For this review, take the finished solid that the model builds, in its own axes (mm). A direction names the side the tool comes from. Round coordinates to 2 decimals unless told otherwise and drop trailing zeros. Loops run counter-clockwise (first coordinate to the right, second up) from the corner with the lowest first, then second, coordinate; pieces in that order, holes last. Notation, with made-up numbers: M 85,-19 L 92,-19 A21 ccw 92,8 Z; hole C -20,-22.75 d2. An arc over 180 degrees is marked long. One line per question, with ' | ' between items. Start each with the question number.
1) For probe 1 along Z at (x, y) = (12.5, -78); probe 2 along X at (y, z) = (-47, -13.5); probe 3 along Z at (x, y) = (29.15, -15.24), list the stretches that pass through material, from the lowest coordinate up. Write a range as from..to.
2) For pin 1 Ø1.1 at (x, y) = (1, -43.5) entering from +Z; pin 2 Ø3 at (y, z) = (-70, -25.5) entering from +X; pin 3 Ø3 at (x, z) = (15.5, 2) entering from -Y; pin 4 Ø13.5 at (x, y) = (18.5, -23) entering from -Z, all flat-tipped, find the tip position at first contact; note any pin that passes through.
3) We need section B-B (y = -15.24). Give the boundary of the cut face in (x, z).
4) We need section D-D (y = -70). Give the boundary of the cut face in (x, z), and give its area (3 significant figures).
5) We need section C-C (z = -7). Give the boundary of the cut face in (x, y).
6) Mouldability with a two-part tool opening along X and no side actions: class faces 1 (the face through (2, -36, 0)), 2 (the face through (27.394, -29, -12)), 3 (the face through (28.194, -68, -26)) as pulls with the +X half, pulls with the -X half, needs draft (parallel to the pull), parting line crosses it, or undercut.
7) We need section A-A (y = -52). Give the boundary of the cut face in (x, z), and give its area (3 significant figures).
8) For faces 4 (the face through (29.78, -59.84, -12.36)), 5 (the face through (29.33, -2.85, -21.12)), 6 (the face through (15, -61.345, -12)), 7 (the face through (15, -57.535, -13)), 8 (the face through (16, -88.015, 2)), list the 3-axis set-ups (+Z, -Z, +X, -X, +Y, -Y) from which the entire face can be reached by the end or side of a thin tool; tool diameter is ignored.
```python
from build123d import *

# Parameters (mm, degrees)
BOSS_EXTRUDE1_DEPTH         = 3.81
SKETCH2_W                   = 27.394147034
SKETCH2_H                   = 24.384
BOSS_EXTRUDE2_DEPTH         = 3.81
SKETCH7_W                   = 24.13
SKETCH7_H                   = 61.344873393
BOSS_EXTRUDE3_DEPTH         = 3.81
FILLET1_R                   = 10
FILLET2_R                   = 10
FILLET3_R                   = 5
FILLET4_R                   = 5
SKETCH8_W                   = 24.384
SKETCH8_H                   = 30.48
BOSS_EXTRUDE4_DEPTH         = 3.81
FILLET5_R                   = 5
FILLET6_R                   = 10
FILLET8_R                   = 10
SKETCH9_W                   = 24.384
SKETCH9_H                   = 30.48
BOSS_EXTRUDE5_DEPTH         = 3.81
FILLET9_R                   = 10
FILLET10_R                  = 10
FILLET11_R                  = 5
F_1_4_0_25_DIAMETER_HOLE1_D = 6.35


with BuildPart() as part:
    # Sketch1 → Boss-Extrude1 (new body)
    with BuildSketch(Plane(origin=(0, 0, 0), x_dir=(0, 0, -1), z_dir=(1, 0, 0))):
        with BuildLine():
            Line((10, 0), (14.384, 0))
            ThreePointArc((14.384, 0), (21.455067812, -2.928932188), (24.384, -10))
            Line((24.384, -10), (24.384, -57.534873393))
            Line((24.384, -57.534873393), (0, -57.534873393))
            Line((0, -57.534873393), (0, -10))
            ThreePointArc((0, -10), (2.928932188, -2.928932188), (10, 0))
        make_face()
    extrude(amount=BOSS_EXTRUDE1_DEPTH)

    # Sketch2 → Boss-Extrude2 (add)
    with BuildSketch(Plane(origin=(0, -57.534873393, 0), x_dir=(-1, 0, 0), z_dir=(0, -1, 0))):
        with Locations((-13.697073517, 12.192)):
            Rectangle(SKETCH2_W, SKETCH2_H)
    extrude(amount=BOSS_EXTRUDE2_DEPTH)

    # Sketch7 → Boss-Extrude3 (add)
    with BuildSketch(Plane(origin=(27.394147034, 0, 0), x_dir=(0, 0, -1), z_dir=(1, 0, 0))):
        with Locations((12.065, -30.672436697)):
            Rectangle(SKETCH7_W, SKETCH7_H)
    extrude(amount=BOSS_EXTRUDE3_DEPTH)

    # Fillet1
    fillet1_edges = [part.edges().sort_by_distance(p)[0] for p in [
        (29.299147034, 0, -24.13),
    ]]
    fillet(fillet1_edges, radius=FILLET1_R)

    # Fillet2
    fillet2_edges = [part.edges().sort_by_distance(p)[0] for p in [
        (29.299147034, 0, 0),
    ]]
    fillet(fillet2_edges, radius=FILLET2_R)

    # Fillet3
    fillet3_edges = [part.edges().sort_by_distance(p)[0] for p in [
        (31.204147034, -61.344873393, -12.065),
    ]]
    fillet(fillet3_edges, radius=FILLET3_R)

    # Fillet4
    fillet4_edges = [part.edges().sort_by_distance(p)[0] for p in [
        (0, -61.344873393, -12.192),
    ]]
    fillet(fillet4_edges, radius=FILLET4_R)

    # Sketch8 → Boss-Extrude4 (add)
    with BuildSketch(Plane(origin=(0, 0, -24.384), x_dir=(-1, 0, 0), z_dir=(0, 0, -1))):
        with Locations((-16.002, -72.933007505)):
            Rectangle(SKETCH8_W, SKETCH8_H)
    extrude(amount=BOSS_EXTRUDE4_DEPTH)

    # Fillet5
    # the kernel refuses this fillet: 5 mm, written as the material it takes off along each edge
    with BuildSketch(Plane(origin=(-8.330814429, -57.693007505, -28.194), x_dir=(0, 0, 1), z_dir=(1, 0, 0))) as fillet5_piece_1:
        with BuildLine():
            CenterArc((5, 4.856325772), FILLET5_R, 180, 76.231471248)
            Line((0, 4.856325772), (-0.1, 4.856325772))
            Line((-0.1, 4.856325772), (-0.1, 0))
            Line((-0.1, 0), (0, -0.1))
            ThreePointArc((0, -0.1), (1.905, -0.1), (3.7862, -0.097126515))
            Line((3.7862, -0.097126515), (3.81, 0))
        make_face()
    extrude(amount=48.665628858, mode=Mode.SUBTRACT)

    # Fillet6
    fillet6_edges = [part.edges().sort_by_distance(p)[0] for p in [
        (3.81, -88.173007505, -26.289),
    ]]
    fillet(fillet6_edges, radius=FILLET6_R)

    # Fillet8
    fillet8_edges = [part.edges().sort_by_distance(p)[0] for p in [
        (28.194, -88.173007505, -26.289),
    ]]
    fillet(fillet8_edges, radius=FILLET8_R)

    # Sketch9 → Boss-Extrude5 (add)
    with BuildSketch(Plane.XY):
        with Locations((16.002, -72.774873393)):
            Rectangle(SKETCH9_W, SKETCH9_H)
    extrude(amount=BOSS_EXTRUDE5_DEPTH)

    # Fillet9
    fillet9_edges = [part.edges().sort_by_distance(p)[0] for p in [
        (3.81, -88.014873393, 1.905),
    ]]
    fillet(fillet9_edges, radius=FILLET9_R)

    # Fillet10
    fillet10_edges = [part.edges().sort_by_distance(p)[0] for p in [
        (28.194, -88.014873393, 1.905),
    ]]
    fillet(fillet10_edges, radius=FILLET10_R)

    # Fillet11
    # the kernel refuses this fillet: 5 mm, written as the material it takes off along each edge
    with BuildSketch(Plane(origin=(3.81, -57.534873393, 3.81), x_dir=(0, -1, 0), z_dir=(1, 0, 0))) as fillet11_piece_1_section:
        with BuildLine():
            CenterArc((FILLET11_R, FILLET11_R), FILLET11_R, 180, 90)
            Line((0, FILLET11_R), (0, 0))
            Line((0, 0), (FILLET11_R, 0))
        make_face()
    fillet11_piece_1 = extrude(amount=36.884, mode=Mode.PRIVATE)
    fillet11_piece_1 = split(fillet11_piece_1, bisect_by=Plane(origin=(27.394147034, -58.779272815, 2.781917075), z_dir=(-1, 0, 0)), keep=Keep.TOP, mode=Mode.PRIVATE)
    add(fillet11_piece_1, mode=Mode.SUBTRACT)
    with BuildSketch(Plane(origin=(-8.69, -57.534873393, 3.81), x_dir=(0, -1, 0), z_dir=(1, 0, 0))) as fillet11_piece_2_section:
        with BuildLine():
            CenterArc((FILLET11_R, FILLET11_R), FILLET11_R, 180, 90)
            Line((0, FILLET11_R), (0, 0))
            Line((0, 0), (FILLET11_R, 0))
        make_face()
    fillet11_piece_2 = extrude(amount=49.384, mode=Mode.PRIVATE)
    fillet11_piece_2 = split(fillet11_piece_2, bisect_by=Plane(origin=(27.831342884, -61.431899575, 0), z_dir=(0, 0, 1)), keep=Keep.TOP, mode=Mode.PRIVATE)
    add(fillet11_piece_2, mode=Mode.SUBTRACT)

    # 1/4 (0.25) Diameter Hole1 (through all)
    with Locations(Plane(origin=(0, -15.24, -12.192), x_dir=(0, 0, -1), z_dir=(-1, 0, 0))):
        with Locations((0, 0)):
            Hole(F_1_4_0_25_DIAMETER_HOLE1_D / 2)


solid = part.part
```
Answers below:
1) probe 1: -28.19..-24.38, 0..3.81 | probe 2: 0..3.81, 27.39..31.2 | probe 3: -24.13..-15.37, -9.02..0
2) pin 1: z = 0 | pin 2: x = 28.19 | pin 3: y = -88.01 | pin 4: through
3) outline: M 0,-24.38 L 3.81,-24.38 L 3.81,-15.37 L 0,-15.37 Z; M 0,-9.02 L 3.81,-9.02 L 3.81,0 L 0,0 Z; M 27.39,-24.13 L 31.2,-24.13 L 31.2,-15.37 L 27.39,-15.37 Z; M 27.39,-9.02 L 31.2,-9.02 L 31.2,0 L 27.39,0 Z
4) outline: M 3.81,-28.19 L 28.19,-28.19 L 28.19,-24.38 L 3.81,-24.38 Z; M 3.81,0 L 28.19,0 L 28.19,3.81 L 3.81,3.81 Z | area: 186 mm^2
5) outline: M 0,-56.34 A5 ccw 5,-61.34 L 26.2,-61.34 A5 ccw 31.2,-56.34 L 31.2,-0.46 L 27.39,-0.46 L 27.39,-57.53 L 3.81,-57.53 L 3.81,-0.46 L 0,-0.46 Z
6) face 1: needs draft | face 2: undercut | face 3: pulls with the +X half
7) outline: M 0,-24.38 L 3.81,-24.38 L 3.81,0 L 0,0 Z; M 27.39,-24.13 L 31.2,-24.13 L 31.2,0 L 27.39,0 Z | area: 185 mm^2
8) face 4: +X, -Y | face 5: -Z, +X, +Y | face 6: +X, -X, -Y | face 7: +Z, -Z, +Y | face 8: +Z, +X, -X, -Y
